```python
from build123d import *

# Parameters (mm, degrees)
SKETCH6_R          = 0.8
CUT_EXTRUDE1_DEPTH = 10
CUT_EXTRUDE2_DEPTH = 10


with BuildPart() as part:
    # Sketch1 → Revolve1 (revolve)
    with BuildSketch(Plane.XY, mode=Mode.PRIVATE) as revolve1_sk:
        Polygon((0, 10.25), (0, 6.5), (2.6, 6.5), (2.6, 5), (4.6, 5), (4.6, 6.281355932), (14.65, 6.281355932), (14.65, 10.25), (13.25, 10.25), (13.25, 8.6), (1.4, 8.6), (1.4, 10.25), align=None)
    revolve(revolve1_sk.sketch.rotate(Axis((0, 0, 0), (1, 0, 0)), 90), axis=Axis((0, 0, 0), (1, 0, 0)))



with BuildPart() as body_2:
    # Sketch3 → Revolve2 (revolve)
    with BuildSketch(Plane.XY, mode=Mode.PRIVATE) as revolve2_sk:
        Polygon((1.094302339, 0), (1.094302339, 3.76292134), (5.013797074, 1.5), (16.794302339, 1.5), (16.794302339, 0), align=None)
    revolve(revolve2_sk.sketch.rotate(Axis((0, 0, 0), (1, 0, 0)), 90), axis=Axis((0, 0, 0), (1, 0, 0)))

    # Sketch6 → Cut-Extrude1 (cut)
    with BuildSketch(Plane(origin=(16.794302339, 0, 0), x_dir=(0, 0, -1), z_dir=(1, 0, 0))):
        Circle(SKETCH6_R)
    extrude(amount=-CUT_EXTRUDE1_DEPTH, mode=Mode.SUBTRACT)


with BuildPart() as part_1:
    add(part.part)

    add(body_2.part)  # Revolve3 merges body 2
    # Sketch8 → Revolve3 (revolve)
    with BuildSketch(Plane.XY, mode=Mode.PRIVATE) as revolve3_sk:
        Polygon((0, 0), (0, 5), (2.6, 6.5), (2.6, 4.723965443), (1.094302339, 3.854650493), (1.094302339, 0), align=None)
    revolve(revolve3_sk.sketch.rotate(Axis((0, 0, 0), (1, 0, 0)), 90), axis=Axis((0, 0, 0), (1, 0, 0)))

    # Sketch9 → Cut-Extrude2 (cut)
    with BuildSketch(Plane.ZY):
        with BuildLine():
            Line((1.060952343, 2), (-1.060952343, 2))
            Line((-1.060952343, 2), (-2.811396527, 4.086098145))
            ThreePointArc((-2.811396527, 4.086098145), (0, 4.959853676), (2.811396527, 4.086098145))
            Line((2.811396527, 4.086098145), (1.060952343, 2))
        make_face()
        with BuildLine():
            Line((2, 1.060952343), (4.086098145, 2.811396527))
            ThreePointArc((4.086098145, 2.811396527), (4.959853676, 0), (4.086098145, -2.811396527))
            Line((4.086098145, -2.811396527), (2, -1.060952343))
            Line((2, -1.060952343), (2, 1.060952343))
        make_face()
        with BuildLine():
            Line((1.060952343, -2), (2.811396527, -4.086098145))
            ThreePointArc((2.811396527, -4.086098145), (0, -4.959853676), (-2.811396527, -4.086098145))
            Line((-2.811396527, -4.086098145), (-1.060952343, -2))
            Line((-1.060952343, -2), (1.060952343, -2))
        make_face()
        with BuildLine():
            Line((-2, -1.060952343), (-4.086098145, -2.811396527))
            ThreePointArc((-4.086098145, -2.811396527), (-4.959853676, 0), (-4.086098145, 2.811396527))
            Line((-4.086098145, 2.811396527), (-2, 1.060952343))
            Line((-2, 1.060952343), (-2, -1.060952343))
        make_face()
    extrude(amount=-CUT_EXTRUDE2_DEPTH, mode=Mode.SUBTRACT)


solid = part_1.part
```
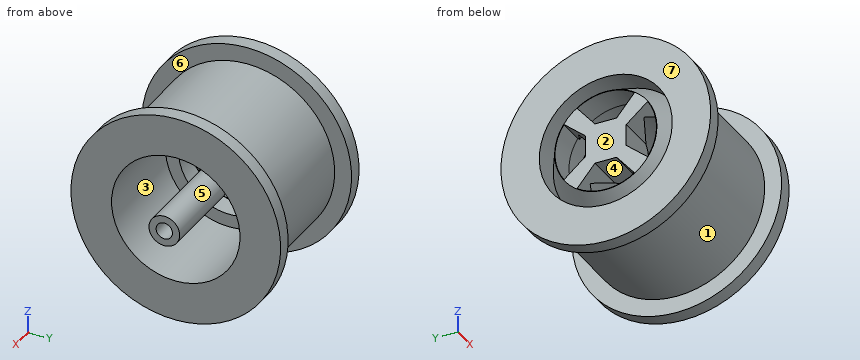
Could you check a few things on this model? Use its own coordinates, in mm. Face numbers are marked on the shaded views. A direction names the side the tool comes from. Coordinates: 2 decimals unless noted, no trailing zeros. Loops run counter-clockwise (first coordinate to the right, second up) from the corner with the lowest first, then second, coordinate; pieces in that order, holes last. Notation, with made-up numbers: M -14,52 L 25,52 A20 cw 25,67 Z; hole C -7,-2.5 d4. An arc over 180 degrees is marked long. Put each result on its own line as item: value. Start each with the question number.
(1) I need wall thicknesses on line 1 (Y direction, x = 3.3, z = 0); line 2 (Y direction, x = 12.5, z = 0); line 3 (X direction, y = -3.5, z = 9.25). Which ranges of each line are inside material? Lowest first, please. Write a range as from..to.
(2) Suppose I cut it at A-A on x = 11.5. Please give me the cut outline in (y, z), then the cut area to 3 significant figures.
(3) Suppose I cut it at C-C on z = 0. Count the separate pieces of the cut face and the enclosed holes in it, then the cut area to 3 significant figures.
(4) Thinking about a two-plate mould opening in X: for the marked faces 1, 2 and 3, which applies, pulls with the +X half, pulls with the -X half, needs draft (parallel to the pull), parting line crosses it, or undercut?
(5) Will these pins go through, and if not, where does the flat tip stop? P1, Ø1, axis at y = 3, z = -2.5, coming from the +X side; P2, Ø10, axis at x = 12.5, z = -4.5, coming from the -Y side; P3, Ø6, axis at x = 9.5, z = -3, coming from the +Y side; P4, Ø0.6, axis at y = 2.5, z = 3, coming from the +X side.
(6) For the marked faces 4, 5, 6 and 7, which set-ups out of +Z, -Z, +X, -X, +Y, -Y let a thin tool reach every point of the face, with its end or its side?
(7) Suppose I cut it at B-B on x = 3. Please give me the cut outline in (y, z).
Solutions:
1. line 1: y = -8.6..-5, -2..2, 5..8.6
1. line 2: y = -8.6..-6.28, -1.5..-0.8, 0.8..1.5, 6.28..8.6
1. line 3: x = 0..1.4, 13.25..14.65
2. outline: C 0,0 d17.2; C 0,0 d3; hole C 0,0 d12.56; hole C 0,0 d1.6
2. area: 113 mm2
3. separate pieces: 3
3. enclosed holes: 0
3. area: 124 mm2
4. face 1: undercut
4. face 2: pulls with the -X half
4. face 3: needs draft
5. P1: stops at x = 2.05
5. P2: stops at y = -10.25
5. P3: stops at y = 8.6
5. P4: stops at x = 1.7
6. face 4: +X, -X
6. face 5: +X
6. face 6: none
6. face 7: +Z, -Z, -X, +Y, -Y
7. outline: C 0,0 d17.2; M -2.31,-1.32 A2.66 ccw -1.32,-2.31 L -1.06,-2 L 1.06,-2 L 1.32,-2.31 A2.66 ccw 2.31,-1.32 L 2,-1.06 L 2,1.06 L 2.31,1.32 A2.66 ccw 1.32,2.31 L 1.06,2 L -1.06,2 L -1.32,2.31 A2.66 ccw -2.31,1.32 L -2,1.06 L -2,-1.06 Z; hole C 0,0 d10
